Here's the drawing with two shaded views (mm, measured from the low corner). I have some questions. A direction names the side the tool comes from. Round coordinates to 2 decimals unless told otherwise and drop trailing zeros. Loops run counter-clockwise (first coordinate to the right, second up) from the corner with the lowest first, then second, coordinate; pieces in that order, holes last. Notation, with made-up numbers: M 8,6 L 35,6 A25 cw 35,41 Z; hole C -25.5,67 d8. An arc over 180 degrees is marked long. One line per item, written item: value. Start each with the question number.
Q1. Imagine slicing it at D-D (x = 13.5). Please give me the cut outline in (y, z), then the cut area to 3 significant figures.
Q2. I'm going to push flat-ended pins straight in: pin 1 Ø5 at (x, z) = (8, 90) entering from +Y; pin 2 Ø1 at (y, z) = (7.5, 53) entering from +X; pin 3 Ø0.8 at (x, y) = (5.5, 0.5) entering from +Z. Where does each tip first touch, or does it pass through?
Q3. Imagine slicing it at A-A (x = 8). Please give me the cut outline in (y, z).
Q4. Imagine slicing it at C-C (z = 35). Please give me the cut outline in (x, y).
Q5. Which directions (+Z, -Z, +X, -X, +Y, -Y) give clear straight access to the entire face, cutting with the end or side of a thin tool? Please do the marked faces 1 and 2.
Q6. Imagine slicing it at B-B (z = 10). Please give me the cut outline in (x, y).
Q7. Please list where these lines run through material, in increasing order: line 1 along Z through (x, y) = (8, 0.6); line 2 along X through (y, z) = (3, 97); line 3 along X through (y, z) = (0.5, 90).
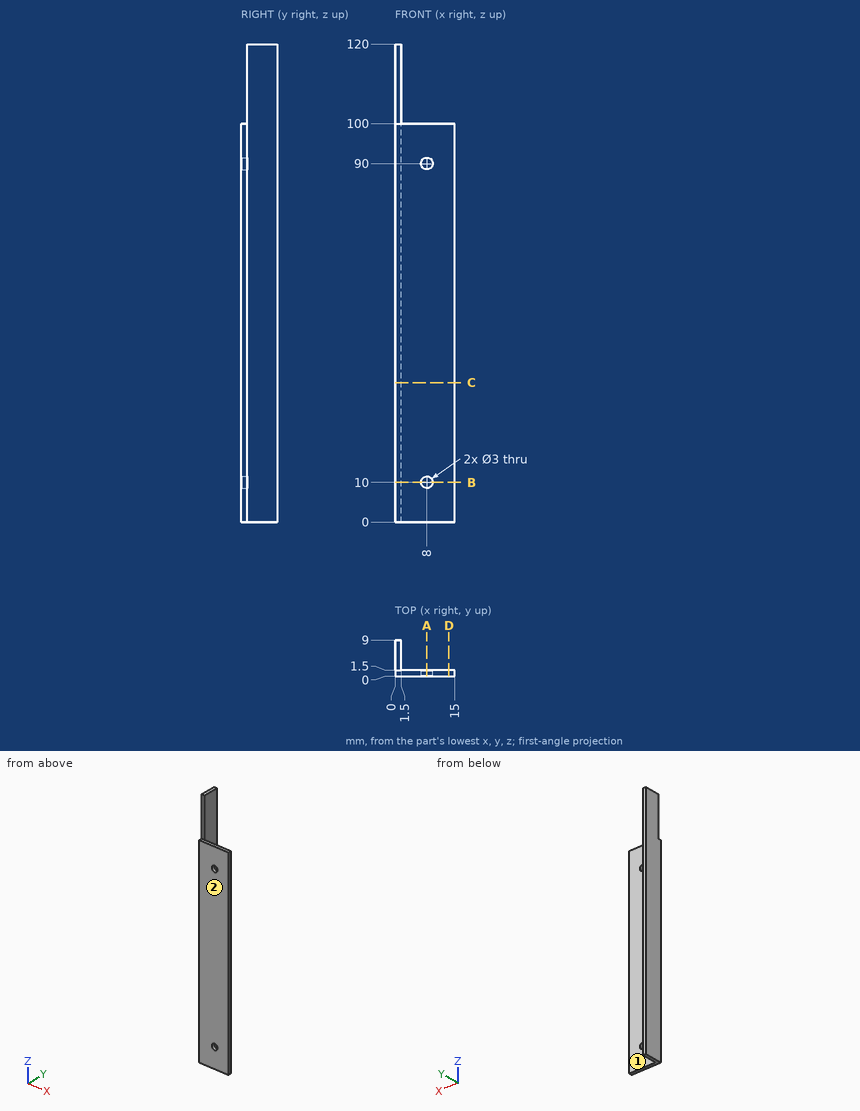
Report:
1. outline: M 0,0 L 1.5,0 L 1.5,100 L 0,100 Z
1. area: 150 mm²
2. pin 1: stops at y = 1.5
2. pin 2: stops at x = 1.5
2. pin 3: stops at z = 100
3. outline: M 0,0 L 1.5,0 L 1.5,8.5 L 0,8.5 Z; M 0,11.5 L 1.5,11.5 L 1.5,88.5 L 0,88.5 Z; M 0,91.5 L 1.5,91.5 L 1.5,100 L 0,100 Z
4. outline: M 0,0 L 15,0 L 15,1.5 L 1.5,1.5 L 1.5,9 L 0,9 Z
5. face 1: +Z, -Z, +X, +Y
5. face 2: +Z, -Z, +X, -X, -Y
6. outline: M 0,0 L 6.5,0 L 6.5,1.5 L 1.5,1.5 L 1.5,9 L 0,9 Z; M 9.5,0 L 15,0 L 15,1.5 L 9.5,1.5 Z
7. line 1: z = 0 to 8.5, 11.5 to 88.5, 91.5 to 100
7. line 2: x = 0 to 1.5
7. line 3: x = 0 to 6.5, 9.5 to 15
